Could you check a few things on this model? Use its own coordinates, in mm. A direction names the side the tool comes from. Round coordinates to 2 decimals unless told otherwise and drop trailing zeros. Loops run counter-clockwise (first coordinate to the right, second up) from the corner with the lowest first, then second, coordinate; pieces in that order, holes last.
from build123d import *

# Parameters (mm, degrees)
F0_W     = 11.0125
F0_H     = 22.325812
F1_DEPTH = 6.0034
F3_DEPTH = 6.0034
F4_W     = 5.50625
F4_H     = 1.8034
F5_DEPTH = 19.05
F6_DEPTH = 19.05


with BuildPart() as f1:
    # F0 (on Top) → F1 (new body)
    with BuildSketch(Plane.XY):
        with Locations((0.79375, 0.028664)):
            Rectangle(F0_W, F0_H)
        with BuildLine():
            Line((-4.7125, 11.19157), (6.3, 11.19157))
            ThreePointArc((6.3, 11.19157), (0.79375, 20.865498), (-4.7125, 11.19157))
        make_face()
    extrude(amount=F1_DEPTH)

    # F2 (on face) → F3 (cut, through all)
    with BuildSketch(Plane.XY.offset(6.0034)):
        with BuildLine():
            ThreePointArc((0.79375, -0.294792), (-1.6637, -2.752242), (0.79375, -5.209692))
            Line((0.79375, -5.209692), (0.79375, -0.294792))
        make_face()
        with BuildLine():
            Line((0.79375, -0.294792), (0.79375, -5.209692))
            ThreePointArc((0.79375, -5.209692), (2.53143, -4.489922), (3.2512, -2.752242))
            ThreePointArc((3.2512, -2.752242), (2.53143, -1.014563), (0.79375, -0.294792))
        make_face()
    extrude(amount=-F3_DEPTH, mode=Mode.SUBTRACT)

    # F4 (on face) → F5 (cut)
    with BuildSketch(Plane.XZ.offset(11.134242)):
        Polygon((-1.9185, 0), (-4.7125, 1.76), (-4.7125, 0), align=None)
        Polygon((6.3, 0), (6.3, 1.76), (3.506, 0), align=None)
        with Locations((-1.959375, 5.1017)):
            Rectangle(F4_W, F4_H)
        with Locations((3.546875, 5.1017)):
            Rectangle(F4_W, F4_H)
    extrude(amount=-F5_DEPTH, mode=Mode.SUBTRACT)

    # F4 (on face) → F6 (cut)
    with BuildSketch(Plane.XZ.offset(11.134242)):
        Polygon((-1.9185, 0), (-4.7125, 1.76), (-4.7125, 0), align=None)
        Polygon((6.3, 0), (6.3, 1.76), (3.506, 0), align=None)
        with Locations((-1.959375, 5.1017)):
            Rectangle(F4_W, F4_H)
        with Locations((3.546875, 5.1017)):
            Rectangle(F4_W, F4_H)
    extrude(amount=-F6_DEPTH, mode=Mode.SUBTRACT)


solid = f1.part
Item 1: If I drill on line 1 along X through (y, z) = (9, 0.5); line 2 along Z through (x, y) = (0, 3.5); line 3 along Y through (x, z) = (2, 3.25), over which ranges is the centre line in solid material (lowest first)?
Results list:
line 1: x = -4.71 to 6.3
line 2: z = 0 to 4.2
line 3: y = -11.13 to -4.89, -0.61 to 20.75
Item 2: If we section it at B-B, the plane x = 2: Please give me the cut outline in (y, z), then the cut area to 3 significant figures.
Results list:
outline: (-11.13, 0) - (-4.89, 0) - (-4.89, 4.2) - (-11.13, 4.2) - close; (-0.61, 0) - (20.75, 0) - (20.75, 6) - (7.92, 6) - (7.92, 4.2) - (-0.61, 4.2) - close
area: 139 mm2
Item 3: For faces 1 (the flat face through (-3.3, -1.74, 0.87)), 2 (the flat face through (1, 7.916, 5)), 3 (the flat face through (6, 7.916, 1)), which set-ups out of +Z, -Z, +X, -X, +Y, -Y let a thin tool reach every point of the face, with its end or its side?
Results list:
face 1: -Z, -X, -Y
face 2: +Z, +X, -X, -Y
face 3: -Z, +X, -Y
Item 4: If we section it at C-C, the plane y = -6.5: Please give me the cut outline in (x, z), then the cut area to 3 significant figures.
Results list:
outline: (-4.71, 1.76) - (-1.92, 0) - (3.51, 0) - (6.3, 1.76) - (6.3, 4.2) - (-4.71, 4.2) - close
area: 41.3 mm2
Item 5: Will these pins go through, and if not, where does the flat tip stop? pin 1 (0.5 mm diameter, centred on x = -1.5, z = 5.5, fed in from -Y); pin 2 (1.5 mm diameter, centred on y = 9, z = 4, fed in from +X); pin 3 (3 mm diameter, centred on y = -7, z = 2.5, fed in from -X).
Results list:
pin 1: stops at y = 7.92
pin 2: stops at x = 6.3
pin 3: stops at x = -4.71
Item 6: If we section it at D-D, the plane x = -1: Please give me the cut outline in (y, z), then the cut area to 3 significant figures.
Results list:
outline: (-11.13, 0) - (-4.43, 0) - (-4.43, 4.2) - (-11.13, 4.2) - close; (-1.07, 0) - (20.61, 0) - (20.61, 6) - (7.92, 6) - (7.92, 4.2) - (-1.07, 4.2) - close
area: 142 mm2
Item 7: If we section it at A-A, the plane z = 3.25: Please give me the cut outline in (x, y).
Results list:
outline: (-4.71, -11.13) - (6.3, -11.13) - (6.3, 11.19) arc R6.4 ccw (long way) to (-4.71, 11.19) - close; hole (0.79, -5.21) arc R2.46 ccw to (3.25, -2.75) arc R2.46 ccw (long way) to start
